The listing builds one solid part. Answer for the finished solid, in the listing's coordinates (mm). Face numbers are marked on the shaded views. A direction names the side the tool comes from. Give positions to 0.01 mm unless a question says otherwise; leave off trailing zeros. Loops run counter-clockwise (first coordinate to the right, second up) from the corner with the lowest first, then second, coordinate; pieces in that order, holes last. Notation, with made-up numbers: M 22,17 L 46,17 A8 cw 46,30 Z; hole C 27,28.5 d7. An arc over 180 degrees is marked long. One line per item, written item: value. Start each with the question number.
Q1. Consider L1, parallel to Z at x = 48, y = 3.5; L2, parallel to X at y = 2, z = -0.5. Determine where each line is inside the solid, lowest interval first.
Q2. A cutting plane is placed at A-A, the plane z = -3. Determine the outline of the cut face in (x, y).
Q3. A cutting plane is placed at C-C, the plane x = 43.5. Determine the outline of the cut face in (y, z), and give its area (3 significant figures).
Q4. A cutting plane is placed at B-B, the plane y = -3. Determine the outline of the cut face in (x, z), and give its area (3 significant figures).
Q5. For the marked faces 1, 2 and 3, determine the directions among +Z, -Z, +X, -X, +Y, -Y from which every point of the face is accessible in a straight line to the end or side of a thin tool.
Q6. Flat-ended cylindrical pins translate along their axes: pin 1 (2 mm diameter, centred on x = 59.5, y = 2.5, fed in from -Z); pin 2 (3.5 mm diameter, centred on x = 54, z = 1.5, fed in from -Y); pin 3 (2.5 mm diameter, centred on y = 3.5, z = -2, fed in from -X). Find the tip coordinate at first contact, or state that the pin passes through.
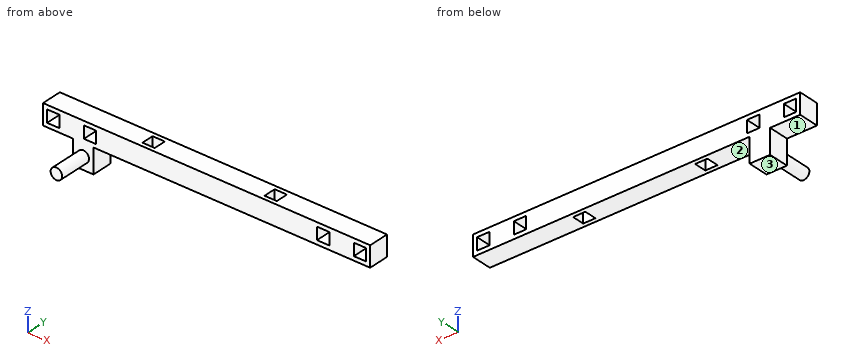
from build123d import *

# Parameters (mm, degrees)
SKETCH1_W           = 80
SKETCH1_H           = 5
SKETCH1_W_2         = 3
SKETCH1_H_2         = 3
BOSS_EXTRUDE1_DEPTH = 5
SKETCH2_W           = 3
SKETCH2_H           = 3
CUT_EXTRUDE1_DEPTH  = 5
SKETCH3_W           = 5
SKETCH3_H           = 5
BOSS_EXTRUDE2_DEPTH = 6
SKETCH4_R           = 1.4
BOSS_EXTRUDE3_DEPTH = 8


with BuildPart() as part:
    # Sketch1 → Boss-Extrude1 (new body)
    with BuildSketch(Plane.XY):
        with Locations((40, 2.5)):
            Rectangle(SKETCH1_W, SKETCH1_H)
        with Locations((54.85, 2.5)):
            Rectangle(SKETCH1_W_2, SKETCH1_H_2, mode=Mode.SUBTRACT)
        with Locations((25, 2.5)):
            Rectangle(SKETCH1_W_2, SKETCH1_H_2, mode=Mode.SUBTRACT)
    extrude(amount=BOSS_EXTRUDE1_DEPTH)

    # Sketch2 → Cut-Extrude1 (cut)
    with BuildSketch(Plane(origin=(0, 5, 0), x_dir=(1, 0, 0), z_dir=(0, 1, 0))):
        with Locations((77.5, -2.5)):
            Rectangle(SKETCH2_W, SKETCH2_H)
        with Locations((2.5, -2.5)):
            Rectangle(SKETCH2_W, SKETCH2_H)
        with Locations((11.5, -2.5)):
            Rectangle(SKETCH2_W, SKETCH2_H)
        with Locations((68.5, -2.5)):
            Rectangle(SKETCH2_W, SKETCH2_H)
    extrude(amount=-CUT_EXTRUDE1_DEPTH, mode=Mode.SUBTRACT)

    # Sketch3 → Boss-Extrude2 (add)
    with BuildSketch(Plane(origin=(0, 0, 0), x_dir=(-1, 0, 0), z_dir=(0, 0, -1))):
        with Locations((-9.85, 2.5)):
            Rectangle(SKETCH3_W, SKETCH3_H)
    extrude(amount=BOSS_EXTRUDE2_DEPTH)

    # Sketch4 → Boss-Extrude3 (add)
    with BuildSketch(Plane.XZ):
        with Locations(Location((9.85, -3, 0), (0, 0, 90))):
            Circle(SKETCH4_R)
    extrude(amount=BOSS_EXTRUDE3_DEPTH)


solid = part.part
Answer block:
1. L1: 0 to 5
1. L2: 7.35 to 12.35
2. outline: M 7.35,0 L 8.45,0 L 8.45,-8 L 11.25,-8 L 11.25,0 L 12.35,0 L 12.35,5 L 7.35,5 Z
3. outline: M 0,0 L 5,0 L 5,5 L 0,5 Z
3. area: 25.0 mm^2
4. outline: C 9.85,-3 d2.8
4. area: 6.16 mm^2
5. face 1: -Z, -X, +Y, -Y
5. face 2: -Z, +X, +Y, -Y
5. face 3: -Z, +X, -X, +Y, -Y
6. pin 1: z = 0
6. pin 2: y = 0
6. pin 3: x = 7.35
